Could you check a few things on this drawing? It's one solid part, dimensions in mm from its lowest x, y, z. A direction names the side the tool comes from. Give positions to 0.01 mm unless a question says otherwise; leave off trailing zeros. Order: outer loops, then holes, each group sorted by start corner. A loop starts at its lowest first (then second) coordinate and runs counter-clockwise, first axis right, second up.
(1) Will these pins go through, and if not, where does the flat tip stop? pin 1 (2 mm diameter, centred on x = 5.5, y = 38, fed in from -Z); pin 2 (22.5 mm diameter, centred on x = 22, y = 21.5, fed in from -Z); pin 3 (2 mm diameter, centred on x = 7.5, z = 2.5, fed in from +Y); pin 4 (4 mm diameter, centred on y = 39.5, z = 1, fed in from +X).
(2) Imagine slicing it at C-C, the plane z = 4.5. Write out the boundary of the cut face in (x, y).
(3) Imagine slicing it at D-D, the plane x = 6.5. Write out the boundary of the cut face in (y, z).
(4) If I drill on probe 1 along Y at (x, z) = (22.5, 2); probe 2 along Y at (x, z) = (22.5, 5.5); probe 3 along X at (y, z) = (25.5, 4.5), over which ranges is the centre line in solid material (lowest first)?
(5) Imagine slicing it at A-A, the plane y = 22.5. Write out the boundary of the cut face in (x, z), then the cut area to 4 significant figures.
(6) On a 3-axis mill with a long thin cutter (end or side, diameter ignored), from which of +Z, -Z, +X, -X, +Y, -Y can I reach the whole of each face in a straight line? I mean the marked faces 1 and 2. Say none if no direction works.
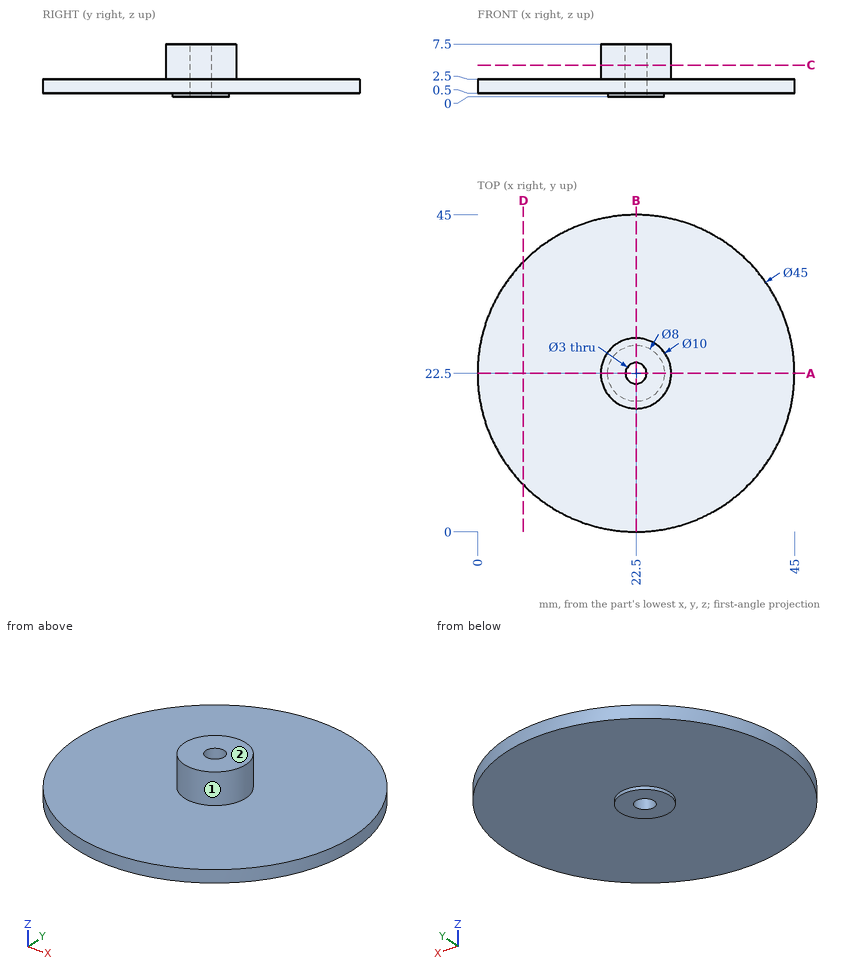
Answer block:
1. pin 1: stops at z = 0.5
1. pin 2: stops at z = 0
1. pin 3: stops at y = 40.11
1. pin 4: stops at x = 39.27
2. outline: circle Ø10 at (22.5, 22.5); hole circle Ø3 at (22.5, 22.5)
3. outline: (6.68, 0.5) - (38.32, 0.5) - (38.32, 2.5) - (6.68, 2.5) - close
4. probe 1: y = 0 to 21, 24 to 45
4. probe 2: y = 17.5 to 21, 24 to 27.5
4. probe 3: x = 18.5 to 26.5
5. outline: (0, 0.5) - (18.5, 0.5) - (18.5, 0) - (21, 0) - (21, 7.5) - (17.5, 7.5) - (17.5, 2.5) - (0, 2.5) - close; (24, 0) - (26.5, 0) - (26.5, 0.5) - (45, 0.5) - (45, 2.5) - (27.5, 2.5) - (27.5, 7.5) - (24, 7.5) - close
5. area: 121.5 mm2
6. face 1: +Z
6. face 2: +Z, +X, -X, +Y, -Y
